```python
from build123d import *

# Parameters (mm, degrees)
SKETCH1_W           = 6
SKETCH1_H           = 2
BOSS_EXTRUDE1_DEPTH = 2
BOSS_EXTRUDE2_DEPTH = 5.5
FILLET1_R           = 1


with BuildPart() as part:
    # Sketch1 → Boss-Extrude1 (new body)
    with BuildSketch(Plane(origin=(0, 0, 0), x_dir=(1, 0, 0), z_dir=(0, 1, 0))):
        Polygon((-14, 5.5), (-14, -5.5), (14, -5.5), (14, 5.5), (5, 5.5), (5, 11.5), (-5, 11.5), (-5, 5.5), align=None)
        with Locations((0, 6.5)):
            Rectangle(SKETCH1_W, SKETCH1_H, mode=Mode.SUBTRACT)
    extrude(amount=BOSS_EXTRUDE1_DEPTH)

    # Sketch2 → Boss-Extrude2 (add, symmetric)
    with BuildSketch(Plane.XY):
        with BuildLine():
            Line((-10.75, -5.929058411), (-10.75, -3.854049622))
            ThreePointArc((-10.75, -3.854049622), (-10, 0), (-9.25, -3.854049622))
            Line((-9.25, -3.854049622), (-9.25, -5.929058411))
            ThreePointArc((-9.25, -5.929058411), (-10, 2), (-10.75, -5.929058411))
        make_face()
        with BuildLine():
            Line((9.25, -5.929058411), (9.25, -3.854049622))
            ThreePointArc((9.25, -3.854049622), (10, 0), (10.75, -3.854049622))
            Line((10.75, -3.854049622), (10.75, -5.929058411))
            ThreePointArc((10.75, -5.929058411), (10, 2), (9.25, -5.929058411))
        make_face()
    extrude(amount=BOSS_EXTRUDE2_DEPTH, both=True)

    # Fillet1
    # the kernel refuses this fillet: 1 mm, written as the material it adds along each edge
    with BuildSketch(Plane(origin=(-6.535898385, 0, -5.5), x_dir=(0.3545926272330996, -0.9350208921259076, 0), z_dir=(0, 0, 1))) as fillet1_piece_1:
        with BuildLine():
            CenterArc((1.443818006, 0.987048159), FILLET1_R, 159.231520484, 101.536959033)
            Line((0.508797114, 1.341640786), (0, 0))
            ThreePointArc((0, 0), (0.641696892, 0.051807363), (1.283393783, 0))
        make_face()
    extrude(amount=11)
    with BuildSketch(Plane(origin=(-13.464101615, 0, -5.5), x_dir=(-1, 0, 0), z_dir=(0, 0, 1))) as fillet1_piece_2:
        with BuildLine():
            CenterArc((1.335898385, 0.6), FILLET1_R, 163.739795292, 53.130102354)
            ThreePointArc((0.375898385, 0.88), (0.214359354, 0.428718708), (0, 0))
            Line((0, 0), (0.535898385, 0))
        make_face()
    extrude(amount=11)
    with BuildSketch(Plane(origin=(13.464101615, 0, -5.5), x_dir=(1, 0, 0), z_dir=(0, 0, 1))) as fillet1_piece_3:
        with BuildLine():
            CenterArc((1.335898385, -0.6), FILLET1_R, 143.130102354, 53.130102354)
            ThreePointArc((0.375898385, -0.88), (0.214359354, -0.428718708), (0, 0))
            Line((0, 0), (0.535898385, 0))
        make_face()
    extrude(amount=11)
    with BuildSketch(Plane(origin=(6.535898385, 0, -5.5), x_dir=(-0.3545926272330986, -0.935020892125908, 0), z_dir=(0, 0, 1))) as fillet1_piece_4:
        with BuildLine():
            CenterArc((1.443818006, -0.987048159), FILLET1_R, 99.231520484, 101.536959033)
            Line((0.508797114, -1.341640786), (0, 0))
            ThreePointArc((0, 0), (0.641696892, -0.051807363), (1.283393783, 0))
        make_face()
    extrude(amount=11)
    # the kernel refuses this fillet: 1 mm, written as the material it takes off along each edge
    with BuildSketch(Plane(origin=(10.75, -5.929058411, 9.808071734), x_dir=(0, 1, 0), z_dir=(0, 0, -1))) as fillet1_2_piece_1:
        with BuildLine():
            CenterArc((1.492359825, 1), FILLET1_R, 144.314665287, 125.685334713)
            ThreePointArc((0.680126963, 1.583333333), (0.253786895, 0.828727108), (0, 0))
            Line((0, 0), (1.492359825, 0))
        make_face()
    extrude(amount=19.616143468, mode=Mode.SUBTRACT)
    with BuildSketch(Plane(origin=(10.75, -3.854049622, -6.956622411), x_dir=(0.8758453103585752, 0.48259195219449225, 0), z_dir=(0, 0, 1))) as fillet1_2_piece_2:
        with BuildLine():
            CenterArc((0.594663609, -0.992902315), FILLET1_R, 96.830510938, 54.314665287)
            Line((-0.281181701, -0.510310363), (0, 0))
            ThreePointArc((0, 0), (0.237865444, -0.014195369), (0.475730887, 0))
        make_face()
    extrude(amount=13.913244822, mode=Mode.SUBTRACT)
    with BuildSketch(Plane(origin=(9.25, -5.929058411, 9.808071734), x_dir=(-0.9188178790368026, 0.39468177708416147, 0), z_dir=(0, 0, -1))) as fillet1_2_piece_3:
        with BuildLine():
            CenterArc((1.507825107, 0.976525112), FILLET1_R, 156.753871206, 125.685334713)
            Line((0.589007228, 1.371206889), (0, 0))
            ThreePointArc((0, 0), (0.861614347, -0.093899551), (1.723228694, 0))
        make_face()
    extrude(amount=19.616143468, mode=Mode.SUBTRACT)
    with BuildSketch(Plane(origin=(9.25, -3.854049622, -6.956622411), x_dir=(0, -1, 0), z_dir=(0, 0, 1))) as fillet1_2_piece_4:
        with BuildLine():
            CenterArc((0.582648964, -1), FILLET1_R, 90, 54.314665287)
            ThreePointArc((-0.229583898, -0.416666667), (-0.102359001, -0.215183904), (0, 0))
            Line((0, 0), (0.582648964, 0))
        make_face()
    extrude(amount=13.913244822, mode=Mode.SUBTRACT)
    with BuildSketch(Plane(origin=(-9.25, -3.854049622, -6.956622411), x_dir=(0, -1, 0), z_dir=(0, 0, 1))) as fillet1_2_piece_5:
        with BuildLine():
            CenterArc((0.582648964, 1), FILLET1_R, 215.685334713, 54.314665287)
            ThreePointArc((-0.229583898, 0.416666667), (-0.102359001, 0.215183904), (0, 0))
            Line((0, 0), (0.582648964, 0))
        make_face()
    extrude(amount=13.913244822, mode=Mode.SUBTRACT)
    with BuildSketch(Plane(origin=(-10.75, -3.854049622, -6.956622411), x_dir=(-0.8758453103585743, 0.4825919521944938, 0), z_dir=(0, 0, 1))) as fillet1_2_piece_6:
        with BuildLine():
            CenterArc((0.594663609, 0.992902315), FILLET1_R, 208.854823775, 54.314665287)
            Line((-0.281181701, 0.510310363), (0, 0))
            ThreePointArc((0, 0), (0.237865444, 0.014195369), (0.475730887, 0))
        make_face()
    extrude(amount=13.913244822, mode=Mode.SUBTRACT)
    with BuildSketch(Plane(origin=(-9.25, -5.929058411, 9.808071734), x_dir=(0.9188178790368028, 0.3946817770841608, 0), z_dir=(0, 0, -1))) as fillet1_2_piece_7:
        with BuildLine():
            CenterArc((1.507825107, -0.976525112), FILLET1_R, 77.560794081, 125.685334713)
            Line((0.589007228, -1.371206889), (0, 0))
            ThreePointArc((0, 0), (0.861614347, 0.093899551), (1.723228694, 0))
        make_face()
    extrude(amount=19.616143468, mode=Mode.SUBTRACT)
    with BuildSketch(Plane(origin=(-10.75, -5.929058411, 9.808071734), x_dir=(0, 1, 0), z_dir=(0, 0, -1))) as fillet1_2_piece_8:
        with BuildLine():
            CenterArc((1.492359825, -1), FILLET1_R, 90, 125.685334713)
            ThreePointArc((0.680126963, -1.583333333), (0.253786895, -0.828727108), (0, 0))
            Line((0, 0), (1.492359825, 0))
        make_face()
    extrude(amount=19.616143468, mode=Mode.SUBTRACT)


solid = part.part
```
Build history of the part. All positions in model axes, mm. A direction names the side the tool comes from. Round coordinates to 2 decimals unless told otherwise and drop trailing zeros. Loops run counter-clockwise (first coordinate to the right, second up) from the corner with the lowest first, then second, coordinate; pieces in that order, holes last.
Item 1: Saw through at B-B (x = -2). List the corners of the cut face in (y, z).
Item 2: Two-plate mould, pull along X, no slides. Class faces 1 (the face through (14, 1, 0)), 2 (the face through (-5, 1, -9)), 3 (the face through (-5.9, -0.4, -0.1)): released by +X, released by -X, zero draft, split by the parting line, or undercut.
Item 3: Saw through at D-D (z = -9). List the corners of the cut face in (x, y).
Item 4: Saw through at A-A (y = 1.25). List the corners of the cut face in (x, z), then the cut area to 3 significant figures.
Item 5: Saw through at C-C (y = -2). List the corners of the cut face in (x, z).
Item 6: Pin check, flat tips, straight feed: P1, Ø2, axis at y = 1, z = -10, coming from the +X side; P2, Ø3.5, axis at x = 10.5, y = -0.5, coming from the -Z side; P3, Ø3, axis at x = -10, y = -2, coming from the +Z side; P4, Ø0.6, axis at y = 1.5, z = -7, coming from the -X side. Stop position of each tip, or through.
Item 7: Which spindle directions (+Z, -Z, +X, -X, +Y, -Y) get a long thin tool onto all of the face, cutting with end or side? Do faces 4 (the face through (0, 0, -3)), 5 (the face through (10, 1, -5.5)), 6 (the face through (0, 1, -5.5)). Say none if no direction does.
Item 8: Drill centre lines: line 1 along X through (y, z) = (-2, 0); line 2 along X through (y, z) = (-1.5, 2); line 3 along Z through (x, y) = (1.5, 0.25). Where is each one in solid material? Low to high.
Worked answers:
1. outline: (0, -11.5) - (2, -11.5) - (2, -7.5) - (0, -7.5) - close; (0, -5.5) - (2, -5.5) - (2, 5.5) - (0, 5.5) - close
2. face 1: released by +X
2. face 2: released by -X
2. face 3: undercut
3. outline: (-5, 0) - (5, 0) - (5, 2) - (-5, 2) - close
4. outline: (-14, -5.5) - (-5, -5.5) - (-5, -11.5) - (5, -11.5) - (5, -5.5) - (14, -5.5) - (14, 5.5) - (-14, 5.5) - close; hole (-3, -7.5) - (3, -7.5) - (3, -5.5) - (-3, -5.5) - close
4. area: 356 mm2
5. outline: (-14, -5.5) - (-12, -5.5) - (-12, 5.5) - (-14, 5.5) - close; (-8, -5.5) - (-6, -5.5) - (-6, 5.5) - (-8, 5.5) - close; (6, -5.5) - (8, -5.5) - (8, 5.5) - (6, 5.5) - close; (12, -5.5) - (14, -5.5) - (14, 5.5) - (12, 5.5) - close
6. P1: stops at x = 5
6. P2: stops at z = -5.5
6. P3: passes through
6. P4: stops at x = -5
7. face 4: +Z, -Z, -Y
7. face 5: -Z, +X, +Y, -Y
7. face 6: +Y, -Y
8. line 1: x = -14 to -12, -8 to -6, 6 to 8, 12 to 14
8. line 2: x = -13.97 to -11.94, -8.06 to -6.03, 6.03 to 8.06, 11.94 to 13.97
8. line 3: z = -11.5 to -7.5, -5.5 to 5.5
